The listing builds one solid part. Answer for the finished solid, in the listing's coordinates (mm). Give positions to 0.01 mm unless a question says otherwise; leave off trailing zeros. Loops run counter-clockwise (first coordinate to the right, second up) from the corner with the lowest first, then second, coordinate; pieces in that order, holes last. Notation, with made-up numbers: (-25, -24) - (-5, -24) arc R14 cw to (-5, -2) - close; hole circle Ø2 at (-19.5, 74.5). An arc over 180 degrees is marked (long way). Answer as CSV lines item,"result". Start each with the question number.
1) Find the intervals of material crossed by line 1 along Z through (x, y) = (-1.3, -0.15); line 2 along Y through (x, z) = (0.35, 5); line 3 along Z through (x, y) = (-0.3, 0.65), in increasing order.
2) Flat-ended cylindrical pins translate along their axes: pin 1 (1.5 mm diameter, centred on y = 1.5, z = 1, fed in from -X); pin 2 (1.1 mm diameter, centred on x = 0.5, y = -0.5, fed in from +Z); pin 3 (1 mm diameter, centred on x = 0, y = 1, fed in from -Z). Find the tip coordinate at first contact, or state that the pin passes through.
3) A cutting plane is placed at A-A (z = -2.5). Determine the outline of the cut face in (x, y).
Autodesk Inventor part; units mm, degrees
ref_plane "YZ Plane" through (0, 0, 0) normal (1, 0, 0) x (0, 1, 0)
ref_plane "XZ Plane" through (0, 0, 0) normal (0, 1, 0) x (-1, 0, 0)
ref_plane "XY Plane" through (0, 0, 0) normal (0, 0, 1) x (1, 0, 0)
sketch "Sketch2" plane through (0, 0, 0) normal (0, 0, 1) x (1, 0, 0)
  circle A0 centre (0, 0) radius 1.25
  dimension "d44" = 2.5
extrude "Extrusion8" add sketch "Sketch2" along normal mid plane 12.5
sketch "Sketch3" plane through (0, 0, 6.25) normal (0, 0, 1) x (1, 0, 0)
  circle A0 centre (0, 0) radius 1.75
  dimension "d47" = 3.5
sketch "Sketch4" plane through (0, 0, 0) normal (0, 1, 0) x (-1, 0, 0)
  line L0 (1.25, 6.25) -> (-1.25, 6.25)
  line L1 (0, 6.25) -> (0, 6.65)
  arc A0 (0, 6.65) -> (-1.761, 6.25) centre (0.2088, 1.6544) ccw
  line L2 (0, 6.25) -> (-1.761, 6.25)
  point P0 (0, 0)
  dimension "d48" = 0.4
  dimension "d49" = 5
revolve "Revolution1" add sketch "Sketch4" angle 360 about axis through (0, 0, 6.25) along (0, 0, 1)
mirror "Mirror1" about plane through (0, 0, 0) normal (0, 0, 1) of "Revolution1"
properties part number "link7" material "Aluminum 6061"
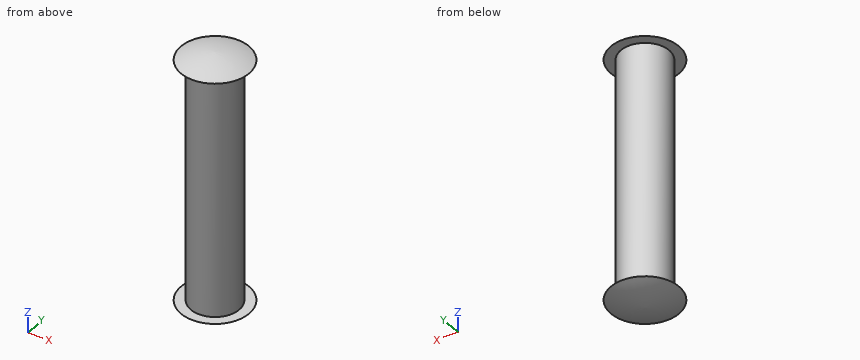
Ans:
1,line 1,"-6.42 to -6.25, 6.25 to 6.42"
1,line 2,"-1.2 to 1.2"
1,line 3,"-6.57 to 6.57"
2,pin 1,"x = -1"
2,pin 2,"z = 6.64"
2,pin 3,"z = -6.6"
3,outline,"circle Ø2.5 at (0, 0)"
